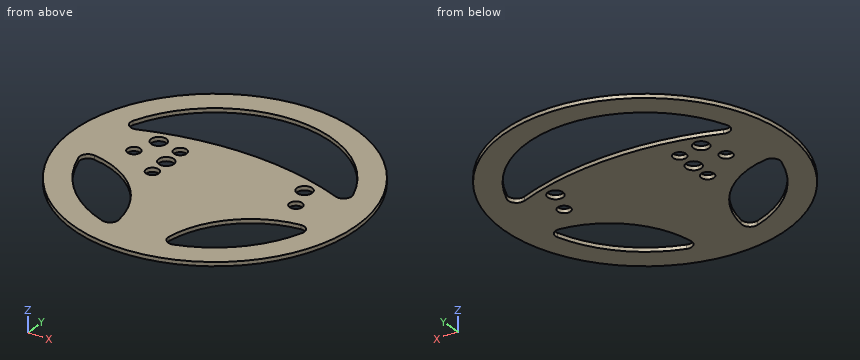
from build123d import *

# Parameters (mm, degrees)
SKETCH1_R           = 111.125
BOSS_EXTRUDE1_DEPTH = 3.175
SKETCH2_R           = 5.999999938
SKETCH2_R_2         = 5.000000033
CUT_EXTRUDE1_DEPTH  = 3.175


with BuildPart() as part:
    # Sketch1 → Boss-Extrude1 (new body)
    with BuildSketch(Plane.XY):
        Circle(SKETCH1_R)
        with BuildLine():
            ThreePointArc((-78.118809332, 23.936541993), (0, 38.1), (78.118809332, 23.936541993))
            ThreePointArc((78.118809332, 23.936541993), (84.832280885, 25.386264259), (86.299834064, 32.095860566))
            ThreePointArc((86.299834064, 32.095860566), (0, 92.075), (-86.299834064, 32.095860566))
            ThreePointArc((-86.299834064, 32.095860566), (-84.832280885, 25.386264259), (-78.118809332, 23.936541993))
        make_face(mode=Mode.SUBTRACT)
        with BuildLine():
            ThreePointArc((19.648389698, -80.882079401), (39.855012865, -39.855012865), (80.882079401, -19.648389698))
            ThreePointArc((80.882079401, -19.648389698), (86.575177486, -21.870616714), (87.75676836, -27.866740606))
            ThreePointArc((87.75676836, -27.866740606), (65.106856878, -65.106856878), (27.866740606, -87.75676836))
            ThreePointArc((27.866740606, -87.75676836), (21.870616714, -86.575177486), (19.648389698, -80.882079401))
        make_face(mode=Mode.SUBTRACT)
        with BuildLine():
            ThreePointArc((-19.648389698, -80.882079401), (-39.855012865, -39.855012865), (-80.882079401, -19.648389698))
            ThreePointArc((-80.882079401, -19.648389698), (-86.575177486, -21.870616714), (-87.75676836, -27.866740606))
            ThreePointArc((-87.75676836, -27.866740606), (-65.106856878, -65.106856878), (-27.866740606, -87.75676836))
            ThreePointArc((-27.866740606, -87.75676836), (-21.870616714, -86.575177486), (-19.648389698, -80.882079401))
        make_face(mode=Mode.SUBTRACT)
    extrude(amount=BOSS_EXTRUDE1_DEPTH)

    # Sketch2 → Cut-Extrude1 (cut)
    with BuildSketch(Plane(origin=(0, 0, 0), x_dir=(-1, 0, 0), z_dir=(0, 0, -1))):
        with Locations((-57.15, 19.05)):
            Circle(SKETCH2_R)
        with Locations((-63.5, 0)):
            Circle(SKETCH2_R_2)
        with Locations((57.15, 19.05)):
            Circle(SKETCH2_R)
        with Locations((63.5, 0)):
            Circle(SKETCH2_R_2)
        with Locations((38.1, 0)):
            Circle(SKETCH2_R)
        with Locations((38.1, 15.875)):
            Circle(SKETCH2_R_2)
        with Locations((38.1, -15.875)):
            Circle(SKETCH2_R_2)
    extrude(amount=-CUT_EXTRUDE1_DEPTH, mode=Mode.SUBTRACT)


solid = part.part
Can you work these out from the model? Positions are in its coordinate system, mm. Give positions to 0.01 mm unless a question says otherwise; leave off trailing zeros. Loops run counter-clockwise (first coordinate to the right, second up) from the corner with the lowest first, then second, coordinate; pieces in that order, holes last. Notation, with made-up numbers: M -7,-34.5 L 39,-34.5 A14 cw 39,-8.5 Z; hole C -4,22 d2. An arc over 180 degrees is marked long. One line per item, written item: value. Start each with the question number.
1) If we section it at B-B, the plane y = 0: Write out the boundary of the cut face in (x, z) (3 decimals), and give its area (3 significant figures).
2) If we section it at D-D, the plane z = 1.7: Give the number of separate pieces and of enclosed holes in the cut face, and give its area (3 significant figures).
3) If we section it at A-A, the plane x = 0: Write out the boundary of the cut face in (y, z) (3 decimals), and give its area (3 significant figures).
4) I'm going to push flat-ended pins straight in: pin 1 (1 mm diameter, centred on x = 2.5, z = 1.5, fed in from +Y); pin 2 (1.5 mm diameter, centred on x = 85, z = 2, fed in from +Y). Where does each tip first touch, or does it pass through?
5) If we section it at C-C, the plane x = -38.1: Write out the boundary of the cut face in (y, z) (3 decimals).
6) If I drill on line 1 (Y direction, x = 63.5, z = 2) (3 decimals); line 2 (Y direction, x = 41, z = 3); line 3 (Y direction, x = 26, z = 1.1), over which ranges is the centre line in solid material (lowest first)? Write a range as [from, to].
Completed:
1. outline: M -111.125,0 L -68.5,0 L -68.5,3.175 L -111.125,3.175 Z; M -58.5,0 L -44.1,0 L -44.1,3.175 L -58.5,3.175 Z; M -32.1,0 L 58.5,0 L 58.5,3.175 L -32.1,3.175 Z; M 68.5,0 L 111.125,0 L 111.125,3.175 L 68.5,3.175 Z
1. area: 604 mm^2
2. separate pieces: 1
2. enclosed holes: 10
2. area: 25,900 mm^2
3. outline: M -111.125,0 L 38.1,0 L 38.1,3.175 L -111.125,3.175 Z; M 92.075,0 L 111.125,0 L 111.125,3.175 L 92.075,3.175 Z
3. area: 534 mm^2
4. pin 1: stops at y = 111.11
4. pin 2: stops at y = 72.46
5. outline: M -104.389,0 L -83.822,0 L -83.822,3.175 L -104.389,3.175 Z; M -41.674,0 L -20.875,0 L -20.875,3.175 L -41.674,3.175 Z; M -10.875,0 L -6,0 L -6,3.175 L -10.875,3.175 Z; M 6,0 L 10.875,0 L 10.875,3.175 L 6,3.175 Z; M 20.875,0 L 34.814,0 L 34.814,3.175 L 20.875,3.175 Z; M 83.822,0 L 104.389,0 L 104.389,3.175 L 83.822,3.175 Z
6. line 1: y = [-91.195, -66.675], [-24.212, -5], [5, 28.847], [66.675, 91.195]
6. line 2: y = [-103.28, -82.44], [-38.74, 34.29], [82.44, 103.28]
6. line 3: y = [-108.04, -88.05], [-59.44, 36.58], [88.33, 108.04]
